Can you work these out from the model? Positions are in its coordinate system, mm. A direction names the side the tool comes from. Round coordinates to 2 decimals unless told otherwise and drop trailing zeros. Write each loop counter-clockwise with the first axis right and the second up, starting at its lowest first coordinate (ties: lowest second). Pieces come first, ordered by that corner, then holes.
Q1. If we section it at D-D (y = 22.5): Please give me the cut outline in (x, z).
Q2. If we section it at A-A (z = 3.05): Please give me the cut outline in (x, y), plus the area to 3 significant figures.
Q3. If we section it at C-C (x = 87): Please give me the cut outline in (y, z).
Q4. I'm going to push flat-ended pins straight in: pin 1 Ø1.5 at (x, y) = (106.5, 27.5) entering from +Z; pin 2 Ø2 at (y, z) = (13.5, 1.5) entering from +X; pin 3 Ø1.6 at (y, z) = (21, 3) entering from +X. Where does each tip first touch, or does it pass through?
Q5. For faces 1 (the flat face through (57, 25, 2)), 2 (the flat face through (58, 0, 2)), which set-ups out of +Z, -Z, +X, -X, +Y, -Y let a thin tool reach every point of the face, with its end or its side?
Q6. If we section it at B-B (y = 16.5): Please give me the cut outline in (x, z), plus the area to 3 significant figures.
Q7. Please list where these lines run through material, in increasing order: line 1 along X through (y, z) = (20, 3.55); line 2 along X through (y, z) = (25, 1.7); line 3 along X through (y, z) = (38, 2.35).
Q8. We'd pull the mould along Y, two halves only. Please class faces 3 (the flat face through (59, 50, 2)), 4 (the flat face through (120, 25, 2)), 5 (the cylindrical face through (135.27, 24.51, 1.97)): +Y half, -Y half, draft (parallel to the pull), parting line (faces both ways), or undercut.
from build123d import *

# Parameters (mm, degrees)
F1_DEPTH = 2
F2_DEPTH = 4


with BuildPart() as f1:
    # F0 (on Top) → F1 (new body)
    with BuildSketch(Plane.XY):
        with BuildLine():
            Line((5, 43), (5, 7))
            ThreePointArc((5, 7), (5.585786, 5.585786), (7, 5))
            Line((7, 5), (108, 5))
            ThreePointArc((108, 5), (109.414214, 5.585786), (110, 7))
            Line((110, 7), (110, 43))
            ThreePointArc((110, 43), (109.414214, 44.414214), (108, 45))
            Line((108, 45), (7, 45))
            ThreePointArc((7, 45), (5.585786, 44.414214), (5, 43))
        make_face()
    extrude(amount=F1_DEPTH)

    # F0 (on Top) → F2 (join)
    with BuildSketch(Plane.XY):
        with BuildLine():
            ThreePointArc((0, 2), (0.585786, 0.585786), (2, 0))
            Line((2, 0), (115, 0))
            Line((115, 0), (115, 50))
            Line((115, 50), (2, 50))
            ThreePointArc((2, 50), (0.585786, 49.414214), (0, 48))
            Line((0, 48), (0, 2))
        make_face()
        with BuildLine():
            ThreePointArc((7, 5), (5.585786, 5.585786), (5, 7))
            Line((5, 7), (5, 43))
            ThreePointArc((5, 43), (5.585786, 44.414214), (7, 45))
            Line((7, 45), (108, 45))
            ThreePointArc((108, 45), (109.414214, 44.414214), (110, 43))
            Line((110, 43), (110, 7))
            ThreePointArc((110, 7), (109.414214, 5.585786), (108, 5))
            Line((108, 5), (7, 5))
        make_face(mode=Mode.SUBTRACT)
        with BuildLine():
            Line((115, 50), (115, 0))
            ThreePointArc((115, 0), (135.275224, 25), (115, 50))
        make_face()
        with BuildLine():
            ThreePointArc((120.000005, 42.797239), (130.27522, 25), (120.000005, 7.202761))
            Line((120.000005, 7.202761), (120.000005, 42.797239))
        make_face(mode=Mode.SUBTRACT)
    extrude(amount=F2_DEPTH)


solid = f1.part
A:
1. outline: (0, 0) - (120, 0) - (120, 4) - (110, 4) - (110, 2) - (5, 2) - (5, 4) - (0, 4) - close; (130.12, 0) - (135.15, 0) - (135.15, 4) - (130.12, 4) - close
2. outline: (0, 2) arc R2 ccw to (2, 0) - (115, 0) arc R25.55 ccw to (115, 50) - (2, 50) arc R2 ccw to (0, 48) - close; hole (5, 7) arc R2 ccw to (7, 5) - (108, 5) arc R2 ccw to (110, 7) - (110, 43) arc R2 ccw to (108, 45) - (7, 45) arc R2 ccw to (5, 43) - close; hole (120, 7.2) arc R20.55 ccw to (120, 42.8) - close
2. area: 2,050 mm2
3. outline: (0, 0) - (50, 0) - (50, 4) - (45, 4) - (45, 2) - (5, 2) - (5, 4) - (0, 4) - close
4. pin 1: stops at z = 2
4. pin 2: stops at x = 133.02
4. pin 3: stops at x = 135.07
5. face 1: +Z
5. face 2: +Z, -Z, +X, -X, -Y
6. outline: (0, 0) - (120, 0) - (120, 4) - (110, 4) - (110, 2) - (5, 2) - (5, 4) - (0, 4) - close; (128.43, 0) - (133.82, 0) - (133.82, 4) - (128.43, 4) - close
6. area: 292 mm2
7. line 1: x = 0 to 5, 110 to 120, 129.66 to 134.78
7. line 2: x = 0 to 120, 130.28 to 135.28
7. line 3: x = 0 to 5, 110 to 120, 125.64 to 131.72
8. face 3: +Y half
8. face 4: undercut
8. face 5: parting line
